```python
from build123d import *

# Parameters (mm, degrees)
SKETCH1_R           = 10
BOSS_EXTRUDE1_DEPTH = 10
BOSS_EXTRUDE1_TAPER = 16.69924423
SKETCH2_R           = 4
CUT_EXTRUDE1_DEPTH  = 7
SKETCH3_R           = 2.5
CUT_EXTRUDE2_DEPTH  = 4.0000001


with BuildPart() as part:
    # Sketch1 → Boss-Extrude1 (new body)
    with BuildSketch(Plane(origin=(0, 0, 0), x_dir=(1, 0, 0), z_dir=(0, 1, 0))):
        Circle(SKETCH1_R)
    extrude(amount=BOSS_EXTRUDE1_DEPTH, taper=BOSS_EXTRUDE1_TAPER)

    # Sketch2 → Cut-Extrude1 (cut)
    with BuildSketch(Plane(origin=(0, 10, 0), x_dir=(1, 0, 0), z_dir=(0, 1, 0))):
        Circle(SKETCH2_R)
    extrude(amount=-CUT_EXTRUDE1_DEPTH, mode=Mode.SUBTRACT)

    # Sketch3 → Cut-Extrude2 (cut, through all)
    with BuildSketch(Plane(origin=(0, 3, 0), x_dir=(1, 0, 0), z_dir=(0, 1, 0))):
        Circle(SKETCH3_R)
    extrude(amount=-CUT_EXTRUDE2_DEPTH, mode=Mode.SUBTRACT)


solid = part.part
```
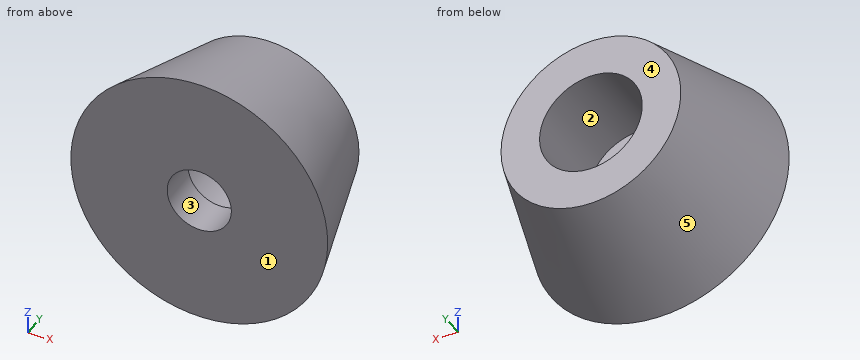
Could you check a few things on this model? Use its own coordinates, in mm. Face numbers are marked on the shaded views. A direction names the side the tool comes from. Round coordinates to 2 decimals unless told otherwise and drop trailing zeros. Loops run counter-clockwise (first coordinate to the right, second up) from the corner with the lowest first, then second, coordinate; pieces in that order, holes last. Notation, with made-up numbers: (2.25, -36.75) -> (39.25, -36.75) arc R20 ccw to (39.25, -28.75) -> close; hole circle Ø6 at (52, 27.25). An arc over 180 degrees is marked (long way). One line per question, with ' | ' between items.
(1) If we section it at A-A on x = 0: List the corners of the cut face in (y, z) for me.
Model answer:
outline: (0, -10) -> (10, -7) -> (10, -4) -> (3, -4) -> (3, -2.5) -> (0, -2.5) -> close; (0, 2.5) -> (3, 2.5) -> (3, 4) -> (10, 4) -> (10, 7) -> (0, 10) -> close
(2) If we section it at C-C on y = 1: List the corners of the cut face in (x, z) for me, and give its area (3 significant figures).
Model answer:
outline: circle Ø19.4 at (0, 0); hole circle Ø5 at (0, 0) | area: 276 mm^2
(3) If I drill on probe 1 along Z at (x, y) = (0, 1.15) (3 decimals); probe 2 along X at (y, z) = (8.25, -2.75); probe 3 along Z at (x, y) = (0, 2.2), over which ranges is the centre line in solid material (lowest first)?
Model answer:
probe 1: z = -9.655 to -2.5, 2.5 to 9.655 | probe 2: x = -7 to -2.9, 2.9 to 7 | probe 3: z = -9.34 to -2.5, 2.5 to 9.34
(4) For pin 1 Ø3 at (x, y) = (4.5, 7.5) entering from -Z; pin 2 Ø6 at (x, z) = (-1.5, 2) entering from +Y; pin 3 Ø2.5 at (x, z) = (0, 2) entering from +Y; pin 4 Ø1.5 at (y, z) = (1, 0.5) entering from -X, each with a flat end and sliding along its axis, tell me the tip position at first contact or that it passes through.
Model answer:
pin 1: stops at z = -7.31 | pin 2: stops at y = 10 | pin 3: stops at y = 3 | pin 4: stops at x = -9.91
(5) For the marked faces 1 and 2, which set-ups out of +Z, -Z, +X, -X, +Y, -Y let a thin tool reach every point of the face, with its end or its side?
Model answer:
face 1: +Z, -Z, +X, -X, -Y | face 2: +Y
(6) If we section it at B-B on y = 6: List the corners of the cut face in (x, z) for me.
Model answer:
outline: circle Ø16.4 at (0, 0); hole circle Ø8 at (0, 0)
(7) Thinking about a two-plate mould opening in X: for the marked faces 3, 4 and 5, which applies, released by +X, released by -X, zero draft, split by the parting line, or undercut?
Model answer:
face 3: undercut | face 4: zero draft | face 5: split by the parting line
